Job drawing, mm, ordinate dimensions from the low corner. One solid piece. Coordinates: 2 decimals unless noted, no trailing zeros. Order: outer loops, then holes, each group sorted by start corner. A loop starts at its lowest first (then second) coordinate and runs counter-clockwise, first axis right, second up. Notation, with made-up numbers: M 2.25,73.5 L 36.25,73.5 A29 cw 36.25,94.5 Z; hole C 21.25,58 d10. An arc over 180 degrees is marked long. Write item = value, one per line. Start each with the question number.
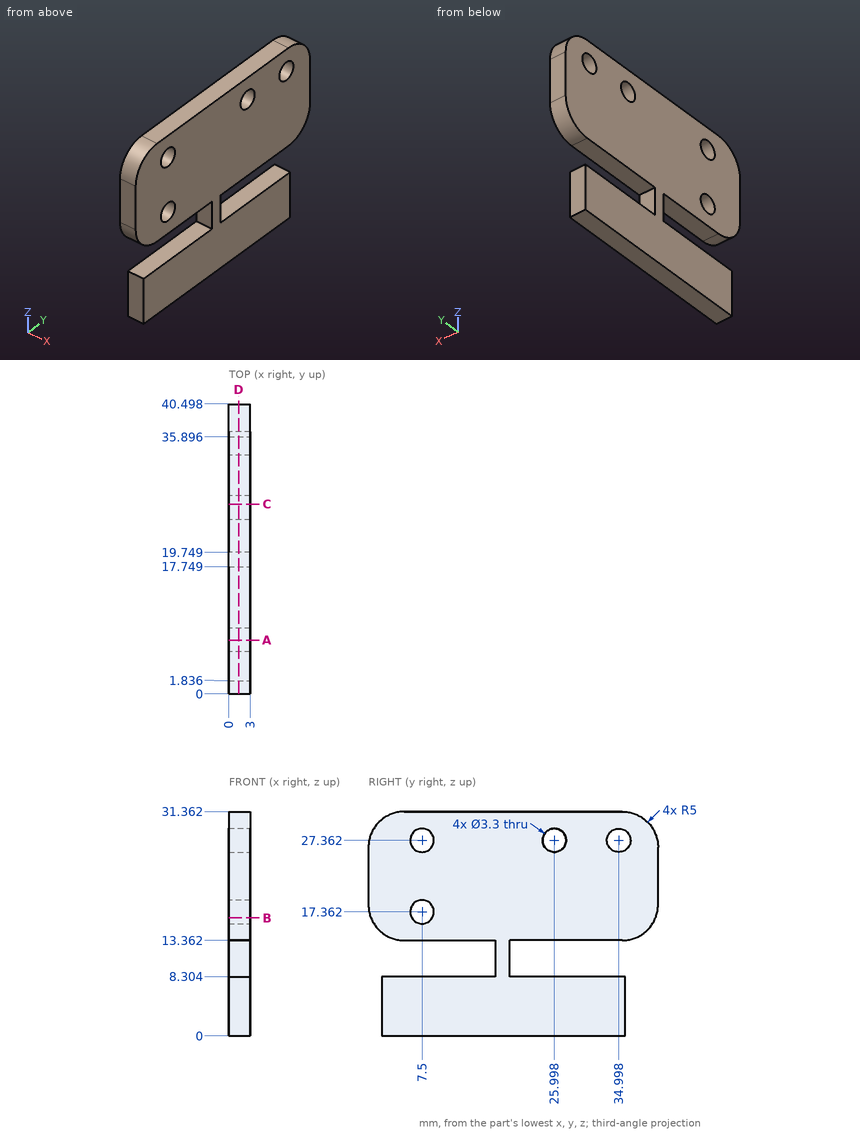
1. Slice it at B-B (z = 16.5). Write the cut outline in (x, y).
2. Slice it at D-D (x = 1.35). Write the cut outline in (y, z), plus the area to 3 significant figures.
3. Slice it at C-C (y = 26.5). Write the cut outline in (x, z), plus the area to 3 significant figures.
4. Slice it at A-A (y = 7.5). Write the cut outline in (x, z).
5. Probe L1, parallel to Z at x = 0.15, y = 23.5; L2, parallel to Z at x = 1.85, y = 25.5 (1 decimal); L3, parallel to Y at x = 1.5, z = 26 (1 decimal). List the from-to ranges inside material, lowest first.
6. Flat gauge pins, fed straight in: pin 1 (4 mm diameter, centred on y = 26, z = 27.36, fed in from -X); pin 2 (1.5 mm diameter, centred on x = 1, z = 5.5, fed in from +Y); pin 3 (1.5 mm diameter, centred on x = 2.5, z = 3.5, fed in from -Y). Where does each tip first touch, or does it go through?
Calculated:
q1.outline = M 0,0.36 L 3,0.36 L 3,6.09 L 0,6.09 Z; M 0,8.91 L 3,8.91 L 3,40.14 L 0,40.14 Z
q2.outline = M 0,18.36 A5 ccw 5,13.36 L 17.75,13.36 L 17.75,8.3 L 1.84,8.3 L 1.84,0 L 35.9,0 L 35.9,8.3 L 19.75,8.3 L 19.75,13.36 L 35.5,13.36 A5 ccw 40.5,18.36 L 40.5,26.36 A5 ccw 35.5,31.36 L 5,31.36 A5 ccw 0,26.36 Z; hole C 7.5,17.36 d3.3; hole C 7.5,27.36 d3.3; hole C 26,27.36 d3.3; hole C 35,27.36 d3.3
q2.area = 966 mm²
q3.outline = M 0,0 L 3,0 L 3,8.3 L 0,8.3 Z; M 0,13.36 L 3,13.36 L 3,25.79 L 0,25.79 Z; M 0,28.93 L 3,28.93 L 3,31.36 L 0,31.36 Z
q3.area = 69.5 mm²
q4.outline = M 0,0 L 3,0 L 3,8.3 L 0,8.3 Z; M 0,13.36 L 3,13.36 L 3,15.71 L 0,15.71 Z; M 0,19.01 L 3,19.01 L 3,25.71 L 0,25.71 Z; M 0,29.01 L 3,29.01 L 3,31.36 L 0,31.36 Z
q5.L1 = 0 to 8.3, 13.36 to 31.36
q5.L2 = 0 to 8.3, 13.4 to 25.8, 28.9 to 31.4
q5.L3 = 0 to 6.6, 8.4 to 25.1, 26.9 to 34.1, 35.9 to 40.5
q6.pin_1 = 0
q6.pin_2 = 35.9
q6.pin_3 = 1.84
